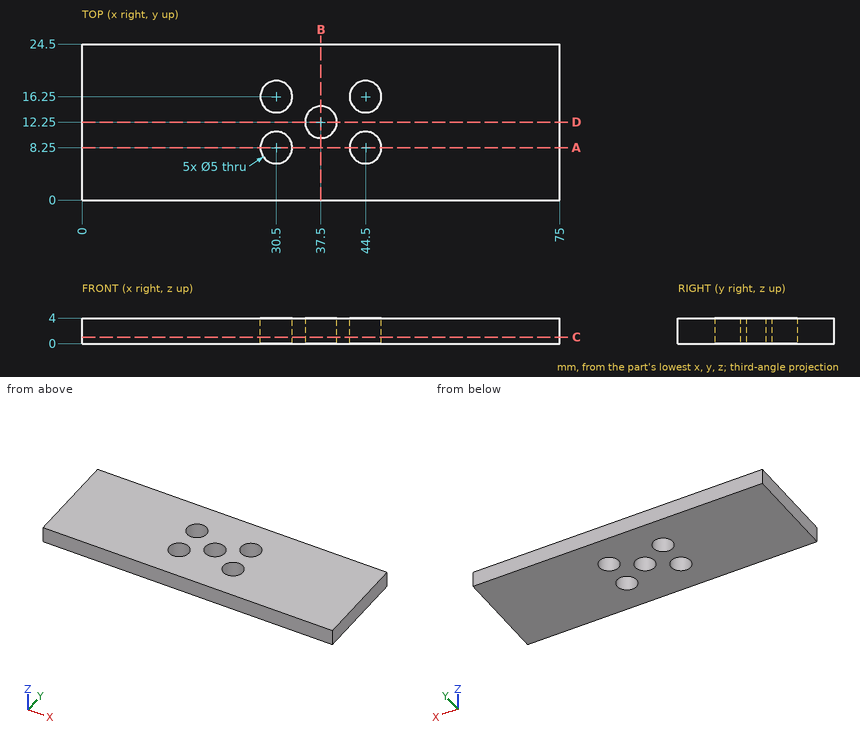
The drawing under review shows one solid part. Ordinate dimensions are in mm from its lowest x, y, z. Coordinates: 2 decimals unless noted, no trailing zeros. Write each loop counter-clockwise with the first axis right and the second up, starting at its lowest first coordinate (ties: lowest second). Pieces come first, ordered by that corner, then holes. Notation, with made-up numbers: M -4,4.25 L 11,4.25 A35 ccw 11,42.25 Z; hole C 49,-3 d11. An arc over 180 degrees is marked long. Put each result on its own line as item: value.
1) Add section C-C on z = 1. Give the boundary of the cut face in (x, y), then the cut area to 3 significant figures.
Computed:
outline: M 0,0 L 75,0 L 75,24.5 L 0,24.5 Z; hole C 30.5,8.25 d5; hole C 30.5,16.25 d5; hole C 37.5,12.25 d5; hole C 44.5,8.25 d5; hole C 44.5,16.25 d5
area: 1,740 mm2
2) Wall thickness on probe 1 along Y at (x, z) = (44.5, 2.4); probe 2 along Y at (x, z) = (37.5, 3.1); probe 3 along Y at (x, z) = (42.5, 3.55): over which ranges is each line inside the solid? List them lowest first. Write a range as [from, to].
Computed:
probe 1: y = [0, 5.75], [10.75, 13.75], [18.75, 24.5]
probe 2: y = [0, 9.75], [14.75, 24.5]
probe 3: y = [0, 6.75], [9.75, 14.75], [17.75, 24.5]
3) Add section A-A on y = 8.25. Give the boundary of the cut face in (x, z).
Computed:
outline: M 0,0 L 28,0 L 28,4 L 0,4 Z; M 33,0 L 42,0 L 42,4 L 33,4 Z; M 47,0 L 75,0 L 75,4 L 47,4 Z
4) Clearance check with flat-ended pins moving along their axes: pin 1 Ø5 at (x, y) = (31.5, 19) entering from -Z; pin 2 Ø3 at (x, y) = (30.5, 8.25) entering from +Z. State where each tip first meets the part, or that it passes through.
Computed:
pin 1: stops at z = 0
pin 2: passes through
5) Add section D-D on y = 12.25. Give the boundary of the cut face in (x, z).
Computed:
outline: M 0,0 L 35,0 L 35,4 L 0,4 Z; M 40,0 L 75,0 L 75,4 L 40,4 Z
6) Add section B-B on x = 37.5. Give the boundary of the cut face in (y, z), then the cut area to 3 significant figures.
Computed:
outline: M 0,0 L 9.75,0 L 9.75,4 L 0,4 Z; M 14.75,0 L 24.5,0 L 24.5,4 L 14.75,4 Z
area: 78.0 mm2
